Build history of the part. All positions in model axes, mm. A direction names the side the tool comes from. Give positions to 0.01 mm unless a question says otherwise; leave off trailing zeros. Loops run counter-clockwise (first coordinate to the right, second up) from the corner with the lowest first, then second, coordinate; pieces in that order, holes last.
1) Band-saw the part on D-D on y = 3.75. List the corners of the cut face in (x, z).
2) Band-saw the part on B-B on z = 1.5. List the corners of the cut face in (x, y), then the cut area to 3 significant figures.
3) Band-saw the part on A-A on x = 14. List the corners of the cut face in (y, z), then the cut area to 3 significant figures.
4) Band-saw the part on C-C on y = 16.25. List the corners of the cut face in (x, z).
5) Wall check: line 1 (Y direction, x = 14, z = 1.2); line 2 (X direction, y = 16.5, z = 18.5); line 3 (Z direction, x = 8.75, y = 56.5). Give the ranges that are in metal, low to high.
6) 3-axis set-ups, long thin cutter, end or side, ignore diameter. For faces 4 (the flat face through (14, 10, 3)), 5 (the flat face through (12, 10, 0)), 6 (the flat face through (10.8, 20, 3.3)), 7 (the cylindrical face through (9.03, 66.11, 13.6)): which of +Z, -Z, +X, -X, +Y, -Y reach the whole face in a straight line?
7) Flat gauge pins, fed straight in: P1, Ø8, axis at y = 37, z = 20, coming from the +X side; P2, Ø1, axis at x = 8, z = 15, coming from the -Y side; P3, Ø3, axis at x = 9, z = 3, coming from the +Y side; P4, Ø8, axis at y = 20.5, z = 6.5, coming from the +X side. Where does each tip first touch, or does it go through?
8) Two-plate mould, pull along Z, no slides. Class faces 1 (the cylindrical face through (9.03, 13.28, 31.15)), 2 (the flat face through (17, 10, 1)), 3 (the cylindrical face through (9.03, 51.4, 17.69)): +Z half, -Z half, draft (parallel to the pull), parting line (faces both ways), or undercut.
```python
from build123d import *

# Parameters (mm, degrees)
SKETCH_1_W          = 17
SKETCH_1_H          = 20
SKETCH_1_R          = 1.5
EXTRUDE_1_DEPTH     = 3
EXTRUDE_2_DEPTH     = 5
SKETCH_4_R          = 1.5
CUT_EXTRUDE_1_DEPTH = 5
FILLET_2_R          = 5
FILLET_3_R          = 1.3
FILLET_4_R          = 10
SKETCH_5_W          = 6
SKETCH_5_H          = 20
CUT_EXTRUDE_2_DEPTH = 10
SKETCH_6_R          = 1.5
CUT_EXTRUDE_3_DEPTH = 1


with BuildPart() as part:
    # 草图1 → 凸台-拉伸1 (new body)
    with BuildSketch(Plane.XY):
        with Locations((8.5, 10)):
            Rectangle(SKETCH_1_W, SKETCH_1_H)
        with Locations((3, 16.25)):
            Circle(SKETCH_1_R, mode=Mode.SUBTRACT)
        with Locations((14, 16.25)):
            Circle(SKETCH_1_R, mode=Mode.SUBTRACT)
        with Locations((14, 3.75)):
            Circle(SKETCH_1_R, mode=Mode.SUBTRACT)
        with Locations((3, 3.75)):
            Circle(SKETCH_1_R, mode=Mode.SUBTRACT)
    extrude(amount=EXTRUDE_1_DEPTH)

    # 草图3 → 凸台-拉伸2 (add)
    with BuildSketch(Plane.ZY.offset(-6)):
        Polygon((3, 20), (10.619084129, 20), (-4.365511909, 61.169839254), (14.428340507, 68.01024212), (34.949549107, 11.628684873), (3, 0), align=None)
    extrude(amount=-EXTRUDE_2_DEPTH)

    # 草图4 → 切除-拉伸1 (cut)
    with BuildSketch(Plane(origin=(11, 0, 0), x_dir=(0, 0, -1), z_dir=(1, 0, 0))):
        with Locations((-16.586518504, 50.385479207)):
            Circle(SKETCH_4_R)
        with Locations((-1.205965334, 57.557548937)):
            Circle(SKETCH_4_R)
    extrude(amount=-CUT_EXTRUDE_1_DEPTH, mode=Mode.SUBTRACT)

    # 圆角2
    fillet_2_edges = [part.edges().sort_by_distance(p)[0] for p in [
        (8.5, 61.169839254, -4.365511909),
        (8.5, 68.01024212, 14.428340507),
    ]]
    fillet(fillet_2_edges, radius=FILLET_2_R)

    # 圆角3
    fillet_3_edges = [part.edges().sort_by_distance(p)[0] for p in [
        (8.5, 20, 10.619084129),
    ]]
    fillet(fillet_3_edges, radius=FILLET_3_R)

    # 圆角4
    fillet_4_edges = [part.edges().sort_by_distance(p)[0] for p in [
        (8.5, 11.628684873, 34.949549107),
    ]]
    fillet(fillet_4_edges, radius=FILLET_4_R)

    # 草图5 → 切除-拉伸2 (cut)
    with BuildSketch(Plane.XY.offset(3)):
        with Locations((3, 10)):
            Rectangle(SKETCH_5_W, SKETCH_5_H)
    extrude(amount=-CUT_EXTRUDE_2_DEPTH, mode=Mode.SUBTRACT)

    # 草图6 → 切除-拉伸3 (cut)
    with BuildSketch(Plane.ZY.offset(-6)):
        with BuildLine():
            Line((3, 0), (25.552622899, 8.20848344))
            ThreePointArc((25.552622899, 8.20848344), (31.195499336, 13.37922703), (31.529347673, 21.025611081))
            Line((31.529347673, 21.025611081), (16.138441224, 63.311779016))
            ThreePointArc((16.138441224, 63.311779016), (13.553069429, 66.133217235), (9.729877403, 66.300141404))
            Line((9.729877403, 66.300141404), (0.332951195, 62.87993997))
            ThreePointArc((0.332951195, 62.87993997), (-2.488487023, 60.294568175), (-2.655411192, 56.47137615))
            Line((-2.655411192, 56.47137615), (9.984092128, 21.744626186))
            ThreePointArc((9.984092128, 21.744626186), (9.827389378, 20.554350633), (8.762491721, 20))
            Line((8.762491721, 20), (0, 20))
            Line((0, 20), (0, 0))
            Line((0, 0), (3, 0))
        make_face()
        with Locations((16.586518504, 50.385479207)):
            Circle(SKETCH_6_R, mode=Mode.SUBTRACT)
        with Locations((1.205965334, 57.557548937)):
            Circle(SKETCH_6_R, mode=Mode.SUBTRACT)
    extrude(amount=-CUT_EXTRUDE_3_DEPTH, mode=Mode.SUBTRACT)


solid = part.part
```
Findings below:
1. outline: (7, 0) - (12.5, 0) - (12.5, 3) - (11, 3) - (11, 13.3) - (7, 13.3) - close; (15.5, 0) - (17, 0) - (17, 3) - (15.5, 3) - close
2. outline: (7, 0) - (17, 0) - (17, 20) - (7, 20) - close; (7, 45.05) - (11, 45.05) - (11, 56.09) - (7, 56.09) - close; (7, 59.03) - (11, 59.03) - (11, 63.3) - (7, 63.3) - close; hole circle Ø3 at (14, 3.75); hole circle Ø3 at (14, 16.25)
2. area: 247 mm2
3. outline: (0, 0) - (2.25, 0) - (2.25, 3) - (0, 3) - close; (5.25, 0) - (14.75, 0) - (14.75, 3) - (5.25, 3) - close; (17.75, 0) - (20, 0) - (20, 3) - (17.75, 3) - close
3. area: 42.0 mm2
4. outline: (7, 0) - (12.5, 0) - (12.5, 3) - (11, 3) - (11, 32.04) - (7, 32.04) - close; (15.5, 0) - (17, 0) - (17, 3) - (15.5, 3) - close
5. line 1: y = 0 to 2.25, 5.25 to 14.75, 17.75 to 20
5. line 2: x = 7 to 11
5. line 3: z = -2.67 to 0.14, 2.27 to 18.62
6. face 4: +Z, +X, +Y, -Y
6. face 5: -Z, +X, -X, -Y
6. face 6: -Z, +X, -X
6. face 7: +X, -X, +Y
7. P1: stops at x = 11
7. P2: stops at y = 4.19
7. P3: stops at y = 64.4
7. P4: stops at x = 17
8. face 1: +Z half
8. face 2: draft
8. face 3: undercut
